```python
from build123d import *

# Parameters (mm, degrees)
F0_W     = 3.893223
F0_H     = 25
F2_DEPTH = 20
F0_W_2   = 26.106777
F3_DEPTH = 5
F4_R     = 2.38125
F5_DEPTH = 25
F6_R     = 6.184118
F7_DEPTH = 6


with BuildPart() as f2:
    # F0 (on Top) → F2 (new body)
    with BuildSketch(Plane.XY):
        with Locations((-11.537091, 4.933417)):
            Rectangle(F0_W, F0_H)
    extrude(amount=F2_DEPTH)

    # F0 (on Top) → F3 (join)
    with BuildSketch(Plane.XY):
        with Locations((-11.537091, 4.933417)):
            Rectangle(F0_W, F0_H)
        with Locations((3.462908, 4.933417)):
            Rectangle(F0_W_2, F0_H)
    extrude(amount=F3_DEPTH)

    # F4 (on face) → F5 (cut)
    with BuildSketch(Plane(origin=(-13.483703, 0, 0), x_dir=(0, -1, 0), z_dir=(-1, 0, 0))):
        with Locations((-4.812612, 12.244398)):
            Circle(F4_R)
    extrude(amount=-F5_DEPTH, mode=Mode.SUBTRACT)

    # F6 (on face) → F7 (cut)
    with BuildSketch(Plane.XY.offset(5)):
        with Locations((6.136364, 4.346591)):
            Circle(F6_R)
    extrude(amount=-F7_DEPTH, mode=Mode.SUBTRACT)


solid = f2.part
```
The listing builds one solid part. Answer for the finished solid, in the listing's coordinates (mm). A direction names the side the tool comes from. Give positions to 0.01 mm unless a question says otherwise; leave off trailing zeros. Order: outer loops, then holes, each group sorted by start corner. A loop starts at its lowest first (then second) coordinate and runs counter-clockwise, first axis right, second up. Notation, with made-up numbers: (33, 21.5) - (71, 21.5) arc R18 cw to (71, 42.5) - close; hole circle Ø6 at (77.25, 41.5). An arc over 180 degrees is marked (long way). Answer in a Markdown table with one row per item. Add a question column.
Q1. The part is cut by section A-A (y = 5.75). Determine the outline of the cut face in (x, z), then the cut area to 3 significant figures.
Q2. The part is cut by section B-B (y = 1.75). Determine the outline of the cut face in (x, z).
Q3. Find the intervals of material crossed by line 1 along X through (y, z) = (2, 12); line 2 along Z through (x, y) = (-4, 14.25); line 3 along Y through (x, z) = (11, 4), in increasing order. Write a range as [from, to].
Q4. The part is cut by section C-C (z = 10.5). Determine the outline of the cut face in (x, y), then the cut area to 3 significant figures.
Q5. The part is cut by section D-D (x = 3.5). Determine the outline of the cut face in (y, z), then the cut area to 3 significant figures.
Q6. For a pull along Y with two mould halves and no side action, classify faces 3 (the flat face through (-12, 5, 20)), 4 (the cylindrical face through (-11.56, 2.54, 12.96)), 5 (the flat face through (-1.9, 17.433, 4.8)), 6 (the flat face through (-1.9, -7.567, 4.8)) as released by +Y, released by -Y, zero draft, split by the parting line, or undercut.
Q7. Given P1, Ø4.5, axis at y = -0.5, z = 16, coming from the +X side; P2, Ø12.5, axis at x = 1, y = 4, coming from the +Z side, each flat-ended and moving along its own axis, determine where each tip first touches the part or whether it passes through.
Q8. Which of the six approach directions +Z, -Z, +X, -X, +Y, -Y give full straight-line access (tool end or side, diameter ignored) to faces 1 (the flat face through (16.516, 5, 2)), 2 (the flat face through (0, 8, 5))?
Determined:
| question | item | result |
|---|---|---|
| 1 | outline | (-13.48, 0) - (0.11, 0) - (0.11, 5) - (-9.59, 5) - (-9.59, 10.06) - (-13.48, 10.06) - close; (-13.48, 14.43) - (-9.59, 14.43) - (-9.59, 20) - (-13.48, 20) - close; (12.16, 0) - (16.52, 0) - (16.52, 5) - (12.16, 5) - close |
| 1 | area | 131 mm² |
| 2 | outline | (-13.48, 0) - (0.52, 0) - (0.52, 5) - (-9.59, 5) - (-9.59, 20) - (-13.48, 20) - close; (11.75, 0) - (16.52, 0) - (16.52, 5) - (11.75, 5) - close |
| 3 | line 1 | x = [-13.48, -9.59] |
| 3 | line 2 | z = [0, 5] |
| 3 | line 3 | y = [-7.57, 0.53], [8.17, 17.43] |
| 4 | outline | (-13.48, -7.57) - (-9.59, -7.57) - (-9.59, 3.19) - (-13.48, 3.19) - close; (-13.48, 6.43) - (-9.59, 6.43) - (-9.59, 17.43) - (-13.48, 17.43) - close |
| 4 | area | 84.7 mm² |
| 5 | outline | (-7.57, 0) - (-1.25, 0) - (-1.25, 5) - (-7.57, 5) - close; (9.94, 0) - (17.43, 0) - (17.43, 5) - (9.94, 5) - close |
| 5 | area | 69.1 mm² |
| 6 | face 3 | zero draft |
| 6 | face 4 | undercut |
| 6 | face 5 | released by +Y |
| 6 | face 6 | released by -Y |
| 7 | P1 | stops at x = -9.59 |
| 7 | P2 | stops at z = 5 |
| 8 | face 1 | +Z, -Z, +X, +Y, -Y |
| 8 | face 2 | +Z, +X, +Y, -Y |
